```python
from build123d import *

# Parameters (mm, degrees)
F2_DEPTH = 50


with BuildPart() as f2:
    # F0 (on Top) → F2 (new body, symmetric)
    with BuildSketch(Plane.XY):
        with BuildLine():
            ThreePointArc((7.5, 6.5), (7.2071067812, 7.2071067812), (6.5, 7.5))
            Line((6.5, 7.5), (2.5, 7.5))
            Line((2.5, 7.5), (3.75, 6.25))
            Line((3.75, 6.25), (3.75, 5))
            Line((3.75, 5), (0, 5))
            Line((0, 5), (0, 2.5))
            ThreePointArc((0, 2.5), (1.767766953, 1.767766953), (2.5, 0))
            Line((2.5, 0), (5, 0))
            Line((5, 0), (5, 3.75))
            Line((5, 3.75), (6.25, 3.75))
            Line((6.25, 3.75), (7.5, 2.5))
            Line((7.5, 2.5), (7.5, 6.5))
        make_face()
    extrude(amount=F2_DEPTH, both=True)

    # F3: F2 across plane


with BuildPart() as f2_1:
    add(f2.part)
    add(f2.part.mirror(Plane.YZ))

    # F4: F2 across plane


with BuildPart() as f2_2:
    add(f2_1.part)
    add(f2_1.part.mirror(Plane.XZ))


solid = f2_2.part
```
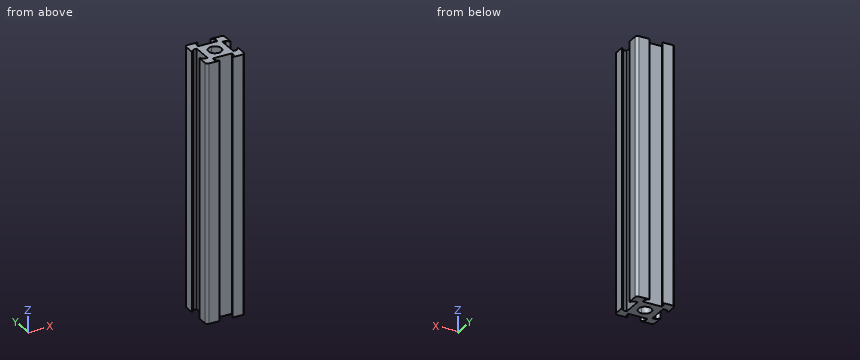
CAD build for the part. Positions are in the model's coordinates, mm. Give positions to 0.01 mm unless a question says otherwise; leave off trailing zeros. Write each loop counter-clockwise with the first axis right and the second up, starting at its lowest first coordinate (ties: lowest second). Pieces come first, ordered by that corner, then holes. Notation, with made-up numbers: M -4.5,39 L 54.5,39 A28 ccw 54.5,72 Z; hole C 46,37.25 d1. An arc over 180 degrees is marked long. Return JSON: item names as keys, results as strings. Group by question number.
(1) Drill centre lines: L1, parallel to Y at x = 3.5, z = 8; L2, parallel to X at y = 0, z = 39.5; L3, parallel to X at y = -5.25, z = -16. Where is each one in solid material? Low to high. Write a range as [from, to].
(2) Band-saw the part on A-A (y = 1.5). Give the cut face in (x, z), and give its area (3 significant figures).
(3) Flat gauge pin, fed straight in: pin 1 Ø4 at (x, z) = (0, 2) entering from +Y. Where does the tip first touch, or does it go through?
Entries:
{
 "1": {"L1": "y = [-7.5, -6.5], [-5, 5], [6.5, 7.5]", "L2": "x = [-5, -2.5], [2.5, 5]", "L3": "x = [-7.5, -3.75], [3.75, 7.5]"},
 "2": {"outline": "M -5,-50 L -2,-50 L -2,50 L -5,50 Z; M 2,-50 L 5,-50 L 5,50 L 2,50 Z", "area": "600 mm^2"},
 "3": {"pin 1": "stops at y = 5"}
}
